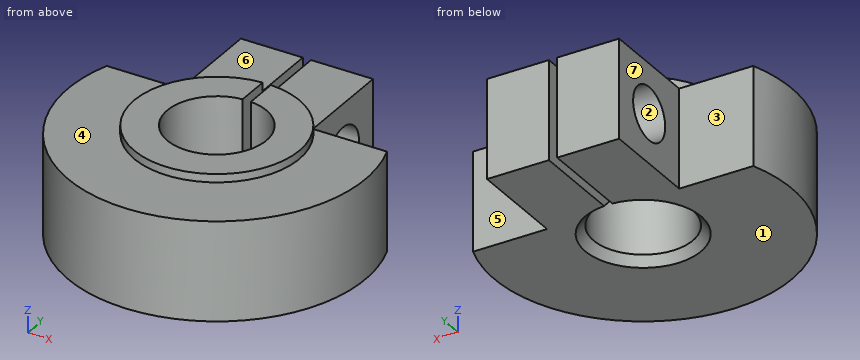
Autodesk Inventor part; units mm, degrees
ref_plane "作業平面1" through (-9, 0, 0) normal (1, 0, 0) x (0, 1, 0)
ref_plane "XZ Plane" through (0, 0, 0) normal (0, 1, 0) x (-1, 0, 0)
ref_plane "XY Plane" through (0, 0, 0) normal (0, 0, 1) x (1, 0, 0)
sketch "スケッチ1" plane through (0, 0, 0) normal (0, 0, 1) x (1, 0, 0)
  circle A0 centre (0, 0) radius 3
  circle A1 centre (0, 0) radius 9
  dimension "d0" = 6
  dimension "d1" = 18
extrude "押し出し1" add sketch "スケッチ1" along normal mid plane 6
ref_plane "作業平面1" through (-9, 0, 0) normal (1, 0, 0) x (0, 1, 0)
sketch "スケッチ5" plane through (0, 0, 3) normal (0, 0, 1) x (1, 0, 0)
  arc A0 (3, 0) -> (3, 0) centre (0, 0) ccw
  circle A1 centre (0, 0) radius 5
  circle A2 centre (0, 0) radius 3
  circle A3 centre (0, 0) radius 3
  dimension "d33" = 10
extrude "押し出し3" add sketch "スケッチ5" along normal blind 0.5
chamfer "面取り3" distance 0.5 angle 45 1 edges at (-3, 0, -3)
sketch "スケッチ10" plane through (0, 0, -3) normal (0, 0, -1) x (-1, 0, 0)
  circle A0 centre (0, 0) radius 9
  line L0 (-9, 9) -> (-4, 9)
  line L1 (-4, 9) -> (-4, 3)
  line L2 (-4, 3) -> (-9, 3)
  line L3 (-9, 3) -> (-9, 9)
  point P0 (-8.4853, 3)
  point P1 (-4, 8.0623)
  dimension "d48" = 4
  dimension "d49" = 6
extrude "押し出し7" cut sketch "スケッチ10" against normal blind 10 contours L1 L2 A0 picked at (-4.4898, 6.0699)
mirror "ミラー4" about plane through (0, 0, 0) normal (1, 0, 0) of "押し出し7"
sketch "スケッチ11" plane through (-4, 3, 3) normal (-1, 0, 0) x (0, 0, 1)
  line L0 (-7.3, -3) -> (1.8, -3)
  line L1 (-6, 0) -> (-6, 5.0623)
  point P0 (-3, -3)
  point P1 (-3, 3)
  dimension "d52" = 6
  dimension "d53" = 3
hole "穴3" at (-4, 6, 0) direction (1, 0, 0) diameter 3.2 end through all
sketch "スケッチ12" plane through (0, 0, -3) normal (0, 0, -1) x (-1, 0, 0)
  line L0 (-4, 8.0623) -> (4, 8.0623)
  line L1 (4, 8.0623) -> (4, 9)
  line L2 (4, 9) -> (-4, 9)
  line L3 (-4, 9) -> (-4, 8.0623)
  arc A0 (4, 8.0623) -> (-4, 8.0623) centre (0, 0) ccw
  point P0 (0, 9)
extrude "押し出し8" add sketch "スケッチ12" against normal up to surface (6 mm away) contours L3 L2 A0 | A0 L2 L1
sketch "スケッチ13" plane through (0, 0, -3) normal (0, 0, -1) x (-1, 0, 0)
  line L0 (-0.25, 9) -> (0.25, 9)
  line L1 (0.25, 9) -> (0.25, 2.9896)
  line L2 (0.25, 2.9896) -> (-0.25, 2.9896)
  line L3 (-0.25, 2.9896) -> (-0.25, 9)
  line L4 (-0.25, 9) -> (0.25, 2.9896) construction
  line L5 (0.25, 9) -> (-0.25, 2.9896) construction
  line L6 (4, 9) -> (-4, 9)
  circle A0 centre (0, 0) radius 3
  point P0 (0, 5.9948)
  point P1 (0, 5.9948)
  dimension "d63" = 0.5
extrude "押し出し9" cut sketch "スケッチ13" against normal blind 10 contours L0 L1 A0 L3
properties part number "shooter_base7" material "ABS プラスチック"
The model under review builds one solid part; all positions refer to its coordinate system, in mm. Face numbers are marked on the shaded views. A direction names the side the tool comes from. Round coordinates to 2 decimals unless told otherwise and drop trailing zeros. Write each loop counter-clockwise with the first axis right and the second up, starting at its lowest first coordinate (ties: lowest second). Pieces come first, ordered by that corner, then holes.
(1) Insertion check: pin 1 (2 mm diameter, centred on x = -6, z = 0.5, fed in from +Y); pin 2 (2 mm diameter, centred on x = -2.5, z = 1.5, fed in from -Y); pin 3 (1.9 mm diameter, centred on y = 6, z = 0, fed in from -X); pin 4 (2 mm diameter, centred on y = -6, z = 0, fed in from -X). Each pin has a flat end and moves straight along its axis. Give the tip position at first contact, or say it passes through.
(2) Machinability: for the marked faces 5, 6 and 7, which of the approach directions +Z, -Z, +X, -X, +Y, -Y give a long, thin tool a straight path to every point of the face, cutting with its end or side? Answer none if there is none.
(3) We need section C-C on y = 6. Give the boundary of the cut face in (x, z), and give its area (3 significant figures).
(4) We need section D-D on x = 0. Give the boundary of the cut face in (y, z), and give its area (3 significant figures).
(5) We need section B-B on y = 0. Give the boundary of the cut face in (x, z), and give its area (4 significant figures).
(6) Wall thickness on L1, parallel to Z at x = 1.6, y = 6; L2, parallel to X at y = 3.5, z = 1.75; L3, parallel to X at y = 0, z = 0.5: over which ranges is each line inside the solid? List them lowest first.
(7) Mouldability with a two-part tool opening along Z and no side actions: class the marked faces 1, 2, 3 and 4 as +Z half, -Z half, draft (parallel to the pull), parting line (faces both ways), or undercut.
(8) We need section A-A on z = 0. Give the boundary of the cut face in (x, y), and give its area (3 significant figures).
Findings below:
1. pin 1: stops at y = 3
1. pin 2: stops at y = -8.87
1. pin 3: passes through
1. pin 4: stops at x = -7.48
2. face 5: +Z, -Z, +X, +Y
2. face 6: +Z, -X, +Y
2. face 7: +Z, -Z, -X, +Y
3. outline: (-4, -3) - (-0.25, -3) - (-0.25, -1.6) - (-4, -1.6) - close; (-4, 1.6) - (-0.25, 1.6) - (-0.25, 3) - (-4, 3) - close; (0.25, -3) - (4, -3) - (4, -1.6) - (0.25, -1.6) - close; (0.25, 1.6) - (4, 1.6) - (4, 3) - (0.25, 3) - close
3. area: 21.0 mm2
4. outline: (-9, -3) - (-3.5, -3) - (-3, -2.5) - (-3, 3.5) - (-5, 3.5) - (-5, 3) - (-9, 3) - close
4. area: 36.9 mm2
5. outline: (-9, -3) - (-3.5, -3) - (-3, -2.5) - (-3, 3.5) - (-5, 3.5) - (-5, 3) - (-9, 3) - close; (3, -2.5) - (3.5, -3) - (9, -3) - (9, 3) - (5, 3) - (5, 3.5) - (3, 3.5) - close
5. area: 73.75 mm2
6. L1: z = -3 to -1.6, 1.6 to 3
6. L2: x = -4 to -0.25, 0.25 to 4
6. L3: x = -9 to -3, 3 to 9
7. face 1: -Z half
7. face 2: undercut
7. face 3: draft
7. face 4: +Z half
8. outline: (-8.49, 3) arc R9 ccw (long way) to (8.49, 3) - (4, 3) - (4, 4.4) - (0.25, 4.4) - (0.25, 2.99) arc R3 cw (long way) to (-0.25, 2.99) - (-0.25, 4.4) - (-4, 4.4) - (-4, 3) - close; (-4, 7.6) - (-0.25, 7.6) - (-0.25, 9) - (-4, 9) - close; (0.25, 7.6) - (4, 7.6) - (4, 9) - (0.25, 9) - close
8. area: 173 mm2
